For this review, take the finished solid that the model builds, in its own axes (mm). Face numbers are marked on the shaded views. A direction names the side the tool comes from. Give positions to 0.01 mm unless a question says otherwise; leave off trailing zeros. Order: outer loops, then holes, each group sorted by start corner. A loop starts at its lowest first (then second) coordinate and runs counter-clockwise, first axis right, second up.
Item 1: Consider section A-A (y = -6.35). Give the boundary of the cut face in (x, z).
Item 2: Consider section C-C (x = 42.5). Give the boundary of the cut face in (y, z), plus the area to 3 significant figures.
Item 3: The part is to be moulded in two halves that separate along Z. For the marked faces 3, 4 and 5, say which applies: released by +Z, released by -Z, zero draft, split by the parting line, or undercut.
Item 4: Machinability: for the marked faces 1 and 2, which of the approach directions +Z, -Z, +X, -X, +Y, -Y give a long, thin tool a straight path to every point of the face, cutting with its end or side? Answer none if there is none.
Item 5: Consider section B-B (z = -24). Give the boundary of the cut face in (x, y), plus the area to 3 significant figures.
Item 6: For probe 1 along Z at (x, y) = (3.5, 6.5); probe 2 along X at (y, z) = (1.25, -14); probe 3 along Z at (x, y) = (35, -6), list the stretches that pass through material, from the lowest coordinate up.
Item 7: For P1, Ø0.6, axis at y = -3, z = -49, coming from the -X side; P2, Ø0.6, axis at y = -7, z = -49, coming from the +X side; P3, Ø1.3, axis at y = 3, z = -49, coming from the +X side, all flat-tipped, find the tip position at first contact; note any pin that passes through.
Item 8: Consider section D-D (y = 3.75). Give the boundary of the cut face in (x, z) (3 decimals).
```python
from build123d import *

# Parameters (mm, degrees)
SKETCH1_W                      = 50.8
SKETCH1_H                      = 1.2192
BASE_FLANGE1_DEPTH             = 12.7
EDGE_FLANGE1_STRIP_W           = 8.6868
EDGE_FLANGE1_STRIP_H           = 1.2192
EDGE_FLANGE1_STRIP_CUT_DEPTH   = 12.7
EDGE_FLANGE1_STRIP_2_W         = 8.6868
EDGE_FLANGE1_STRIP_2_H         = 1.2192
EDGE_FLANGE1_STRIP_CUT_2_DEPTH = 12.7
EDGE_FLANGE1_DEPTH             = 12.7
EDGE_FLANGE1_BEND_DEPTH        = 12.7
EDGE_FLANGE2_STRIP_W           = 8.6868
EDGE_FLANGE2_STRIP_H           = 1.2192
EDGE_FLANGE2_STRIP_CUT_DEPTH   = 12.7
EDGE_FLANGE2_DEPTH             = 12.7
EDGE_FLANGE3_STRIP_W           = 8.6868
EDGE_FLANGE3_STRIP_H           = 1.2192
EDGE_FLANGE3_STRIP_CUT_DEPTH   = 12.7
EDGE_FLANGE3_DEPTH             = 12.7
SKETCH18_W                     = 10.7442
SKETCH18_H                     = 12.7
BOSS_EXTRUDE1_DEPTH            = 1.2192
FILLET1_R                      = 2.54
F_8_CLEARANCE_HOLE1_D          = 4.4958


# Sheet-metal steps are written as plain solids
with BuildPart() as part:
    # Sketch1 → Base-Flange1 (new body)
    with BuildSketch(Plane(origin=(0, 0, 0), x_dir=(1, 0, 0), z_dir=(0, 1, 0))):
        with Locations((25.4, -0.6096)):
            Rectangle(SKETCH1_W, SKETCH1_H)
    extrude(amount=BASE_FLANGE1_DEPTH)

    # Edge-Flange1 strip (across the edge) → Edge-Flange1 strip cut (cut)
    with BuildSketch(Plane(origin=(50.8, 12.7, 0), x_dir=(-1, 0, 0), z_dir=(0, -1, 0))):
        with Locations((-1.2192, -0.6096)):
            Rectangle(EDGE_FLANGE1_STRIP_W, EDGE_FLANGE1_STRIP_H)
    extrude(amount=EDGE_FLANGE1_STRIP_CUT_DEPTH, mode=Mode.SUBTRACT)

    # Edge-Flange1 strip 2 (across the edge) → Edge-Flange1 strip cut 2 (cut)
    with BuildSketch(Plane(origin=(0, 0, 0), x_dir=(1, 0, 0), z_dir=(0, 1, 0))):
        with Locations((-1.2192, -0.6096)):
            Rectangle(EDGE_FLANGE1_STRIP_2_W, EDGE_FLANGE1_STRIP_2_H)
    extrude(amount=EDGE_FLANGE1_STRIP_CUT_2_DEPTH, mode=Mode.SUBTRACT)

    # Edge-Flange1 section (across the edge) → Edge-Flange1 (add)
    with BuildSketch(Plane(origin=(50.8, 12.7, 0), x_dir=(-1, 0, 0), z_dir=(0, -1, 0))):
        with BuildLine():
            Line((0, 1.905), (0, 49.5808))
            Line((0, 49.5808), (1.2192, 49.5808))
            Line((1.2192, 49.5808), (1.2192, 1.905))
            ThreePointArc((1.2192, 1.905), (1.777161582, 0.557961582), (3.1242, 0))
            Line((3.1242, 0), (3.1242, -1.2192))
            ThreePointArc((3.1242, -1.2192), (0.915056994, -0.304143006), (0, 1.905))
        make_face()
    extrude(amount=EDGE_FLANGE1_DEPTH)

    # Edge-Flange1 section 2 (across the edge) → Edge-Flange1 bend (add)
    with BuildSketch(Plane(origin=(0, 0, 0), x_dir=(1, 0, 0), z_dir=(0, 1, 0))):
        with BuildLine():
            Line((0, 1.905), (0, 49.5808))
            Line((0, 49.5808), (1.2192, 49.5808))
            Line((1.2192, 49.5808), (1.2192, 1.905))
            ThreePointArc((1.2192, 1.905), (1.777161582, 0.557961582), (3.1242, 0))
            Line((3.1242, 0), (3.1242, -1.2192))
            ThreePointArc((3.1242, -1.2192), (0.915056994, -0.304143006), (0, 1.905))
        make_face()
    extrude(amount=EDGE_FLANGE1_BEND_DEPTH)

    # Edge-Flange2 strip (across the edge) → Edge-Flange2 strip cut (cut)
    with BuildSketch(Plane(origin=(49.5808, 12.7, -49.5808), x_dir=(0, 0, 1), z_dir=(0, -1, 0))):
        with Locations((-1.2192, -0.6096)):
            Rectangle(EDGE_FLANGE2_STRIP_W, EDGE_FLANGE2_STRIP_H)
    extrude(amount=EDGE_FLANGE2_STRIP_CUT_DEPTH, mode=Mode.SUBTRACT)

    # Edge-Flange2 section (across the edge) → Edge-Flange2 (add)
    with BuildSketch(Plane(origin=(49.5808, 12.7, -49.5808), x_dir=(0, 0, 1), z_dir=(0, -1, 0))):
        with BuildLine():
            Line((0, 1.905), (0, 22.225))
            Line((0, 22.225), (1.2192, 22.225))
            Line((1.2192, 22.225), (1.2192, 1.905))
            ThreePointArc((1.2192, 1.905), (1.777161582, 0.557961582), (3.1242, 0))
            Line((3.1242, 0), (3.1242, -1.2192))
            ThreePointArc((3.1242, -1.2192), (0.915056994, -0.304143006), (0, 1.905))
        make_face()
    extrude(amount=EDGE_FLANGE2_DEPTH)

    # Edge-Flange3 strip (across the edge) → Edge-Flange3 strip cut (cut)
    with BuildSketch(Plane(origin=(1.2192, 0, -49.5808), x_dir=(0, 0, 1), z_dir=(0, 1, 0))):
        with Locations((-1.2192, -0.6096)):
            Rectangle(EDGE_FLANGE3_STRIP_W, EDGE_FLANGE3_STRIP_H)
    extrude(amount=EDGE_FLANGE3_STRIP_CUT_DEPTH, mode=Mode.SUBTRACT)

    # Edge-Flange3 section (across the edge) → Edge-Flange3 (add)
    with BuildSketch(Plane(origin=(1.2192, 0, -49.5808), x_dir=(0, 0, 1), z_dir=(0, 1, 0))):
        with BuildLine():
            Line((0, 1.905), (0, 22.225))
            Line((0, 22.225), (1.2192, 22.225))
            Line((1.2192, 22.225), (1.2192, 1.905))
            ThreePointArc((1.2192, 1.905), (1.777161582, 0.557961582), (3.1242, 0))
            Line((3.1242, 0), (3.1242, -1.2192))
            ThreePointArc((3.1242, -1.2192), (0.915056994, -0.304143006), (0, 1.905))
        make_face()
    extrude(amount=EDGE_FLANGE3_DEPTH)

    # Sketch18 → Boss-Extrude1 (add)
    with BuildSketch(Plane.XY.offset(-48.3616)):
        with Locations((18.0721, -6.35)):
            Rectangle(SKETCH18_W, SKETCH18_H)
        with Locations((32.7279, -6.35)):
            Rectangle(SKETCH18_W, SKETCH18_H)
    extrude(amount=-BOSS_EXTRUDE1_DEPTH)

    # Fillet1
    fillet1_edges = [part.edges().sort_by_distance(p)[0] for p in [
        (23.4442, 12.7, -48.9712),
        (12.7, 0, -48.9712),
        (12.7, -12.7, -48.9712),
        (23.4442, -12.7, -48.9712),
        (38.1, -12.7, -48.9712),
        (38.1, 0, -48.9712),
        (27.3558, -12.7, -48.9712),
        (27.3558, 12.7, -48.9712),
    ]]
    fillet(fillet1_edges, radius=FILLET1_R)

    # #8 Clearance Hole1 (through all)
    with Locations(Plane.XY.offset(-48.3616)):
        with Locations((18.0975, -6.35), (32.7025, -6.35)):
            Hole(F_8_CLEARANCE_HOLE1_D / 2)


solid = part.part
```
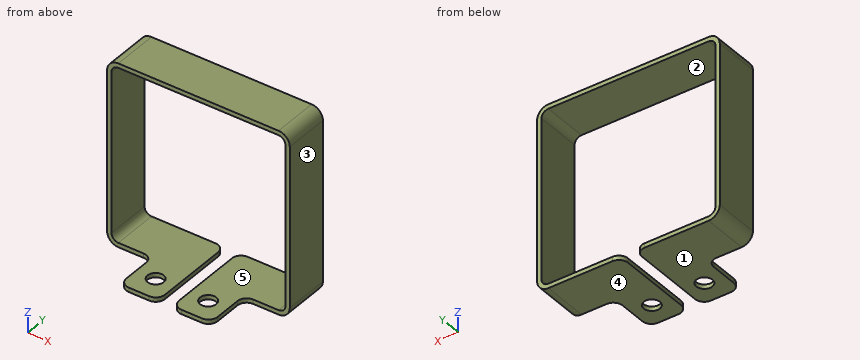
Resolved:
1. outline: (12.7, -49.58) - (15.85, -49.58) - (15.85, -48.36) - (12.7, -48.36) - close; (20.35, -49.58) - (23.44, -49.58) - (23.44, -48.36) - (20.35, -48.36) - close; (27.36, -49.58) - (30.45, -49.58) - (30.45, -48.36) - (27.36, -48.36) - close; (34.95, -49.58) - (38.1, -49.58) - (38.1, -48.36) - (34.95, -48.36) - close
2. outline: (0, -49.58) - (12.7, -49.58) - (12.7, -48.36) - (0, -48.36) - close; (0, 0) - (12.7, 0) - (12.7, 1.22) - (0, 1.22) - close
2. area: 31.0 mm2
3. face 3: zero draft
3. face 4: released by -Z
3. face 5: undercut
4. face 1: -Z, +X, -X, +Y, -Y
4. face 2: +Y, -Y
5. outline: (0, 0) - (1.22, 0) - (1.22, 12.7) - (0, 12.7) - close; (49.58, 0) - (50.8, 0) - (50.8, 12.7) - (49.58, 12.7) - close
5. area: 31.0 mm2
6. probe 1: z = -49.58 to -48.36, 0 to 1.22
6. probe 2: x = 0 to 1.22, 49.58 to 50.8
6. probe 3: z = -49.58 to -48.36
7. P1: stops at x = 12.7
7. P2: stops at x = 38.1
7. P3: stops at x = 50.16
8. outline: (0, -46.457) arc R3.124 ccw to (3.124, -49.581) - (23.444, -49.581) - (23.444, -48.362) - (3.124, -48.362) arc R1.905 cw to (1.219, -46.457) - (1.219, -1.905) arc R1.905 cw to (3.124, 0) - (47.676, 0) arc R1.905 cw to (49.581, -1.905) - (49.581, -46.457) arc R1.905 cw to (47.676, -48.362) - (27.356, -48.362) - (27.356, -49.581) - (47.676, -49.581) arc R3.124 ccw to (50.8, -46.457) - (50.8, -1.905) arc R3.124 ccw to (47.676, 1.219) - (3.124, 1.219) arc R3.124 ccw to (0, -1.905) - close
